For this review, take the finished solid that the model builds, in its own axes (mm). Coordinates: 2 decimals unless noted, no trailing zeros. Order: outer loops, then holes, each group sorted by start corner. A loop starts at its lowest first (then second) coordinate and runs counter-clockwise, first axis right, second up. Notation, with made-up numbers: (24.5, -29) -> (72.5, -29) arc R22 ccw to (72.5, -21) -> close; hole circle Ø9 at (29.5, -9). An arc over 180 degrees is marked (long way). Return JSON: item names as keys, results as strings. Group by question number.
Item 1: For line 1 along X through (y, z) = (0.6, 100.5); line 2 along X through (y, z) = (1.25, 290); line 3 along X through (y, z) = (0.75, 146), list the stretches that pass through material, from the lowest coordinate up.
Item 2: Take a section at A-A (z = 250). Write out the cut boundary in (x, y), then the cut area to 3 significant figures.
Item 3: Take a section at B-B (y = 4.5). Write out the cut boundary in (x, z).
Item 4: Insertion check: pin 1 (6.5 mm diameter, centred on x = 10, z = 290, fed in from +Y); pin 2 (0.6 mm diameter, centred on x = 1, z = 160.5, fed in from +Y). Each pin has a flat end and moves straight along its axis. Give the tip position at first contact, or say it passes through.
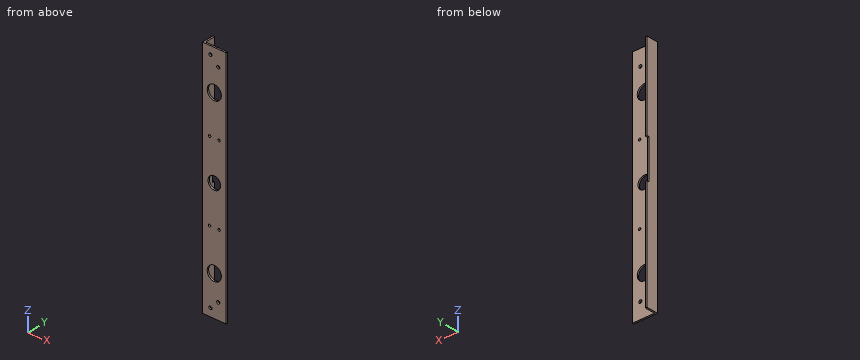
```python
from build123d import *

# Parameters (mm, degrees)
BOSS_EXTRUDE1_DEPTH = 300
SKETCH2_R           = 8
SKETCH2_R_2         = 1.977693409
CUT_EXTRUDE1_DEPTH  = 10
SKETCH3_W           = 300
SKETCH3_H           = 10
CUT_EXTRUDE2_DEPTH  = 10
SKETCH4_W           = 50
SKETCH4_H           = 3
CUT_EXTRUDE3_DEPTH  = 10
SKETCH5_R           = 1.55
CUT_EXTRUDE4_DEPTH  = 273
SKETCH6_R           = 9
CUT_EXTRUDE5_DEPTH  = 5


with BuildPart() as part:
    # Sketch1 → Boss-Extrude1 (new body)
    with BuildSketch(Plane.XY):
        Polygon((0, 0), (0, 25), (2, 25), (2, 2), (30, 2), (30, 0), align=None)
    extrude(amount=BOSS_EXTRUDE1_DEPTH)

    # Sketch2 → Cut-Extrude1 (cut)
    with BuildSketch(Plane(origin=(0, 2, 0), x_dir=(1, 0, 0), z_dir=(0, 1, 0))):
        with Locations(Location((15, -150, 0), (0, 0, 180))):
            Circle(SKETCH2_R)
        with Locations(Location((10, -10, 0), (0, 0, 180))):
            Circle(SKETCH2_R_2)
        with Locations(Location((20, -20, 0), (0, 0, 180))):
            Circle(SKETCH2_R_2)
        with Locations(Location((10, -290, 0), (0, 0, 180))):
            Circle(SKETCH2_R_2)
        with Locations(Location((20, -280, 0), (0, 0, 180))):
            Circle(SKETCH2_R_2)
    extrude(amount=-CUT_EXTRUDE1_DEPTH, mode=Mode.SUBTRACT)

    # Sketch3 → Cut-Extrude2 (cut)
    with BuildSketch(Plane(origin=(2, 0, 0), x_dir=(0, 0, -1), z_dir=(1, 0, 0))):
        with Locations((-150, 20)):
            Rectangle(SKETCH3_W, SKETCH3_H)
    extrude(amount=-CUT_EXTRUDE2_DEPTH, mode=Mode.SUBTRACT)

    # Sketch4 → Cut-Extrude3 (cut)
    with BuildSketch(Plane(origin=(2, 0, 0), x_dir=(0, 0, -1), z_dir=(1, 0, 0))):
        with Locations((-165, 13.5)):
            Rectangle(SKETCH4_W, SKETCH4_H)
    extrude(amount=-CUT_EXTRUDE3_DEPTH, mode=Mode.SUBTRACT)

    # Sketch5 → Cut-Extrude4 (cut)
    with BuildSketch(Plane.XZ):
        with Locations((21, 199.5)):
            Circle(SKETCH5_R)
        with Locations((9, 199.5)):
            Circle(SKETCH5_R)
        with Locations((21, 100.5)):
            Circle(SKETCH5_R)
        with Locations((9, 100.5)):
            Circle(SKETCH5_R)
    extrude(amount=-CUT_EXTRUDE4_DEPTH, mode=Mode.SUBTRACT)

    # Sketch6 → Cut-Extrude5 (cut)
    with BuildSketch(Plane.XZ):
        with Locations((15, 250)):
            Circle(SKETCH6_R)
        with Locations((15, 50)):
            Circle(SKETCH6_R)
        with Locations((-238, 50)):
            Circle(SKETCH6_R)
        with Locations((-238, 250)):
            Circle(SKETCH6_R)
    extrude(amount=-CUT_EXTRUDE5_DEPTH, mode=Mode.SUBTRACT)


solid = part.part
```
Findings below:
{
 "1": {"line 1": "x = 0 to 7.45, 10.55 to 19.45, 22.55 to 30", "line 2": "x = 0 to 8.02, 11.98 to 30", "line 3": "x = 0 to 8.07, 21.93 to 30"},
 "2": {"outline": "(0, 0) -> (6, 0) -> (6, 2) -> (2, 2) -> (2, 15) -> (0, 15) -> close; (24, 0) -> (30, 0) -> (30, 2) -> (24, 2) -> close", "area": "50.0 mm2"},
 "3": {"outline": "(0, 0) -> (2, 0) -> (2, 300) -> (0, 300) -> close"},
 "4": {"pin 1": "stops at y = 2", "pin 2": "stops at y = 12"}
}
